Could you check a few things on this model? Use its own coordinates, in mm. A direction names the side the tool comes from. Give positions to 0.01 mm unless a question says otherwise; leave off trailing zeros. Order: outer loops, then holes, each group sorted by start corner. A loop starts at its lowest first (then second) coordinate and runs counter-clockwise, first axis right, second up. Notation, with made-up numbers: M -12,29.5 L 10,29.5 A20 cw 10,63.5 Z; hole C -3,-3 d6. An arc over 180 degrees is marked long. Use a Markdown table: item, result. Add a question column.
Item 1: Suppose I cut it at D-D on y = -24. Write out the boundary of the cut face in (x, z) (3 decimals), plus the area to 3 significant figures.
Item 2: If I drill on L1, parallel to X at y = -15.5, z = 2.9; L2, parallel to Y at x = 4.5, z = 4.05; L3, parallel to Y at x = -28, z = 2.4, over which ranges is the centre line in solid material (lowest first)? Write a range as from..to.
Item 3: Suppose I cut it at B-B on x = -4.5. Write out the boundary of the cut face in (y, z), plus the area to 3 significant figures.
Item 4: Suppose I cut it at A-A on y = 30.5. Write out the boundary of the cut face in (x, z).
Item 5: Suppose I cut it at C-C on z = 2.8. Count the separate pieces of the cut face and the enclosed holes in it, plus the area to 3 significant figures.
Item 6: I'm going to push flat-ended pins straight in: pin 1 Ø1.5 at (x, z) = (27, 3.5) entering from -Y; pin 2 Ø5.5 at (x, y) = (35.5, 15.5) entering from -Z; pin 3 Ø2.5 at (y, z) = (29.5, 1.5) entering from +X. Where does each tip first touch, or does it pass through?
Item 7: If we mould it in two halves opening along Y, with no side actions, what happens to faces 1 (the face through (-0.719, 23.406, 2.535)), 2 (the face through (-22, -34, 0)), 3 (the face through (37, 16.3, 3.2))? For each: released by +Y, released by -Y, zero draft, split by the parting line, or undercut.
Item 8: For faces 4 (the face through (-38.719, 37.594, 2.535)), 5 (the face through (-24, -25.2, 2.5)), 6 (the face through (-10.757, -23.292, 1.014)), which set-ups out of +Z, -Z, +X, -X, +Y, -Y let a thin tool reach every point of the face, with its end or its side?
from build123d import *

# Parameters (mm, degrees)
ESBO_O1_W                                    = 82
ESBO_O1_H                                    = 80
ESBO_O1_R                                    = 1.5
ESBO_O1_W_2                                  = 8
ESBO_O1_H_2                                  = 24
RESSALTO_EXTRUS_O1_DEPTH                     = 5
CORTE_EXTRUS_O1_DEPTH                        = 92.372862492
ESCAREADO_PARA_PARAFUSO_COM_CABE_A_E_2_COUNT = 2
ESCAREADO_PARA_PARAFUSO_COM_CABE_A_E_2_PITCH = 31
ESCAREADO_PARA_PARAFUSO_COM_CABE_A_E_3_COUNT = 2
ESCAREADO_PARA_PARAFUSO_COM_CABE_A_E_3_PITCH = 43.840620434
ESCAREADO_PARA_PARAFUSO_COM_CABE_A_E_4_COUNT = 2
ESCAREADO_PARA_PARAFUSO_COM_CABE_A_E_4_PITCH = 31
ESBO_O5_R                                    = 11.05
CORTE_EXTRUS_O2_DEPTH                        = 58.497826046
CHANFRO1_SIZE                                = 1
ESBO_O6_W                                    = 44
ESBO_O6_H                                    = 19
CORTE_EXTRUS_O3_DEPTH                        = 10
FILETE1_R                                    = 8
FILETE2_R                                    = 5
ESBO_O7_R                                    = 1.6
CORTE_EXTRUS_O5_DEPTH                        = 58.497826046


with BuildPart() as part:
    # Esboço1 → Ressalto-extrusão1 (new body)
    with BuildSketch(Plane.XY):
        Rectangle(ESBO_O1_W, ESBO_O1_H)
        with Locations((-37, 19.5)):
            Circle(ESBO_O1_R, mode=Mode.SUBTRACT)
        with Locations(Location((-37, -19.5, 0), (0, 0, 180))):
            Circle(ESBO_O1_R, mode=Mode.SUBTRACT)
        with Locations((-19, -19.5)):
            Circle(ESBO_O1_R, mode=Mode.SUBTRACT)
        with Locations(Location((-19, 19.5, 0), (0, 0, 180))):
            Circle(ESBO_O1_R, mode=Mode.SUBTRACT)
        with Locations((-19, 30.5)):
            Circle(ESBO_O1_R, mode=Mode.SUBTRACT)
        with Locations(Location((-37, 30.5, 0), (0, 0, 180))):
            Circle(ESBO_O1_R, mode=Mode.SUBTRACT)
        with Locations((-37, -30.5)):
            Circle(ESBO_O1_R, mode=Mode.SUBTRACT)
        with Locations(Location((-19, -30.5, 0), (0, 0, 180))):
            Circle(ESBO_O1_R, mode=Mode.SUBTRACT)
        with Locations((-28, 25)):
            Rectangle(ESBO_O1_W_2, ESBO_O1_H_2, mode=Mode.SUBTRACT)
        with Locations((-28, -25)):
            Rectangle(ESBO_O1_W_2, ESBO_O1_H_2, mode=Mode.SUBTRACT)
    extrude(amount=RESSALTO_EXTRUS_O1_DEPTH)

    # Esboço2 → Corte-extrusão1 (cut, through all)
    with BuildSketch(Plane(origin=(41, 0, 0), x_dir=(0, 0, -1), z_dir=(1, 0, 0))):
        Polygon((-2, 25), (0, 28.464101615), (0, 21.535898385), align=None)
        Polygon((-2, -25), (0, -21.535898385), (0, -28.464101615), align=None)
    extrude(amount=-CORTE_EXTRUS_O1_DEPTH, mode=Mode.SUBTRACT)

    # Esboço3 → Escareado para parafuso com cabeça escareada elevada de M31 (revolve, cut)
    with BuildSketch(Plane(origin=(35.5, 15.5, 0), x_dir=(0, 1, 0), z_dir=(1, 0, 0))):
        Polygon((0, 0), (0, 5), (1.725, 5), (1.7, 4.975), (1.7, 1.45), (3.15, 0), align=None)
    escareado_para_parafuso_com_cabe_a_escar = revolve(axis=Axis((35.5, 15.5, -6.35), (0, 0, 1)), mode=Mode.SUBTRACT)

    # Escareado para parafuso com cabe_a e 2: Escareado para parafuso com cabeça escareada elevada de M31 ×2
    with Locations(*[(-i * ESCAREADO_PARA_PARAFUSO_COM_CABE_A_E_2_PITCH, 0, 0) for i in range(1, ESCAREADO_PARA_PARAFUSO_COM_CABE_A_E_2_COUNT)]):
        add(escareado_para_parafuso_com_cabe_a_escar, mode=Mode.SUBTRACT)

    # Escareado para parafuso com cabe_a e 3: Escareado para parafuso com cabeça escareada elevada de M31 ×2
    with Locations(*[Vector(-0.7071067811865476, -0.7071067811865476, 0) * (i * ESCAREADO_PARA_PARAFUSO_COM_CABE_A_E_3_PITCH) for i in range(1, ESCAREADO_PARA_PARAFUSO_COM_CABE_A_E_3_COUNT)]):
        add(escareado_para_parafuso_com_cabe_a_escar, mode=Mode.SUBTRACT)

    # Escareado para parafuso com cabe_a e 4: Escareado para parafuso com cabeça escareada elevada de M31 ×2
    with Locations(*[(0, -i * ESCAREADO_PARA_PARAFUSO_COM_CABE_A_E_4_PITCH, 0) for i in range(1, ESCAREADO_PARA_PARAFUSO_COM_CABE_A_E_4_COUNT)]):
        add(escareado_para_parafuso_com_cabe_a_escar, mode=Mode.SUBTRACT)

    # Esboço5 → Corte-extrusão2 (cut, through all)
    with BuildSketch(Plane.XY.offset(5)):
        with Locations((20, 0)):
            Circle(ESBO_O5_R)
    extrude(amount=-CORTE_EXTRUS_O2_DEPTH, mode=Mode.SUBTRACT)

    # Chanfro1
    chanfro1_edges = [part.edges().sort_by_distance(p)[0] for p in [
        (8.95, 0, 0),
        (8.95, 0, 5),
    ]]
    chamfer(chanfro1_edges, length=CHANFRO1_SIZE)

    # Esboço6 → Corte-extrusão3 (cut)
    with BuildSketch(Plane.XY):
        with Locations((19, 30.5)):
            Rectangle(ESBO_O6_W, ESBO_O6_H)
        with Locations((19, -30.5)):
            Rectangle(ESBO_O6_W, ESBO_O6_H)
    extrude(amount=CORTE_EXTRUS_O3_DEPTH, mode=Mode.SUBTRACT)

    # Filete1
    filete1_edges = [part.edges().sort_by_distance(p)[0] for p in [
        (-3, 21, 2.5),
        (-3, -21, 2.5),
        (-3, -40, 2.5),
        (-41, -40, 2.5),
        (-41, 40, 2.5),
        (-3, 40, 2.5),
    ]]
    fillet(filete1_edges, radius=FILETE1_R)

    # Filete2
    filete2_edges = [part.edges().sort_by_distance(p)[0] for p in [
        (41, 21, 2.5),
        (41, -21, 2.5),
    ]]
    fillet(filete2_edges, radius=FILETE2_R)

    # Esboço7 → Corte-extrusão5 (cut, through all)
    with BuildSketch(Plane.XY):
        with Locations((-17.5, 0)):
            Circle(ESBO_O7_R)
        with Locations(Location((-4.5, 0, 0), (0, 0, 180))):
            Circle(ESBO_O7_R)
    extrude(amount=CORTE_EXTRUS_O5_DEPTH, mode=Mode.SUBTRACT)


solid = part.part
Findings below:
| question | item | result |
|---|---|---|
| 1 | outline | M -41,1.423 L -32,1.423 L -32,5 L -41,5 Z; M -24,1.423 L -1.245,1.423 L -1.245,5 L -24,5 Z |
| 1 | area | 114 mm^2 |
| 2 | L1 | x = -41..-32, -24..2.8, 6.2..33.8, 37.2..41 |
| 2 | L2 | y = -21.02..-17.2, -13.8..13.8, 17.2..21.02 |
| 2 | L3 | y = -40..-37, -13..13, 37..40 |
| 3 | outline | M -36.66,0 L -28.46,0 L -25,2 L -21.54,0 L -1.6,0 L -1.6,5 L -36.66,5 Z; M 1.6,0 L 21.54,0 L 25,2 L 28.46,0 L 36.66,0 L 36.66,5 L 1.6,5 Z |
| 3 | area | 337 mm^2 |
| 4 | outline | M -41,0 L -38.5,0 L -38.5,5 L -41,5 Z; M -35.5,0 L -32,0 L -32,5 L -35.5,5 Z; M -24,0 L -20.5,0 L -20.5,5 L -24,5 Z; M -17.5,0 L -3,0 L -3,5 L -17.5,5 Z |
| 5 | separate pieces | 1 |
| 5 | enclosed holes | 17 |
| 5 | area | 3,970 mm^2 |
| 6 | pin 1 | stops at y = -21 |
| 6 | pin 2 | stops at z = 0.4 |
| 6 | pin 3 | stops at x = -2.96 |
| 7 | face 1 | released by +Y |
| 7 | face 2 | zero draft |
| 7 | face 3 | undercut |
| 8 | face 4 | +Z, -Z, -X, +Y |
| 8 | face 5 | +Z, -Z |
| 8 | face 6 | -Z, +X, -X |
